Read the model definition and answer for the solid it produces. Units are mm, in the model's axes. Face numbers are marked on the shaded views. Give positions to 0.01 mm unless a question says otherwise; leave off trailing zeros. Order: outer loops, then holes, each group sorted by start corner. A loop starts at its lowest first (then second) coordinate and runs counter-clockwise, first axis right, second up.
```python
from build123d import *

# Parameters (mm, degrees)
F0_W     = 19.05
F0_H     = 152.4
F1_DEPTH = 6.35
F2_W     = 12.7
F2_H     = 152.4
F3_DEPTH = 5.08
F4_W     = 2.286
F4_H     = 3.81
F5_DEPTH = 152.4


with BuildPart() as f1:
    # F0 (on Top) → F1 (new body)
    with BuildSketch(Plane.XY):
        with Locations((-26.88839, 35.860999)):
            Rectangle(F0_W, F0_H)
    extrude(amount=F1_DEPTH)

    # F2 (on face) → F3 (cut)
    with BuildSketch(Plane.XY.offset(6.35)):
        with Locations((-26.903349, 35.860999)):
            Rectangle(F2_W, F2_H)
    extrude(amount=-F3_DEPTH, mode=Mode.SUBTRACT)

    # F4 (on face) → F5 (cut)
    with BuildSketch(Plane.XZ.offset(40.339001)):
        with Locations((-34.396349, 3.175)):
            Rectangle(F4_W, F4_H)
        with Locations((-19.410349, 3.175)):
            Rectangle(F4_W, F4_H)
    extrude(amount=-F5_DEPTH, mode=Mode.SUBTRACT)


solid = f1.part
```
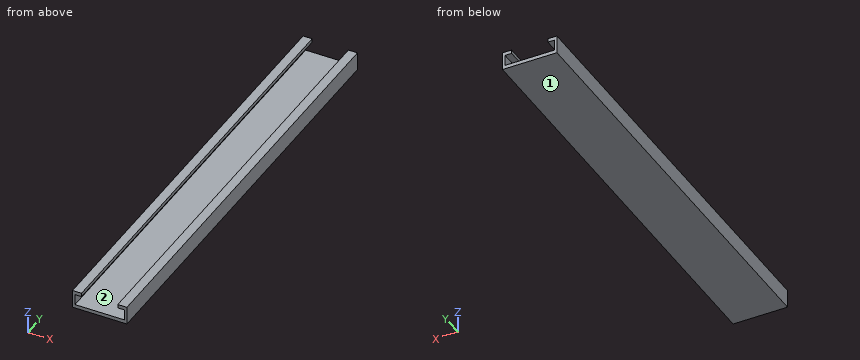
1) The part is cut by section C-C on x = -25.25. Determine the outline of the cut face in (y, z).
Final values:
outline: (-40.34, 0) - (112.06, 0) - (112.06, 1.27) - (-40.34, 1.27) - close
2) Consider L1, parallel to Z at x = -34.75, y = 49.5; L2, parallel to X at y = -12, z = 3.75; L3, parallel to Z at x = -26.25, y = 105. Determine where each line is inside the solid, lowest interval first.
Final values:
L1: z = 0 to 1.27, 5.08 to 6.35
L2: x = -36.41 to -35.54, -18.27 to -17.36
L3: z = 0 to 1.27
3) The part is cut by section B-B on y = 64. Determine the outline of the cut face in (x, z), and give its area (3 significant figures).
Final values:
outline: (-36.41, 0) - (-17.36, 0) - (-17.36, 6.35) - (-20.55, 6.35) - (-20.55, 5.08) - (-18.27, 5.08) - (-18.27, 1.27) - (-35.54, 1.27) - (-35.54, 5.08) - (-33.25, 5.08) - (-33.25, 6.35) - (-36.41, 6.35) - close
area: 39.0 mm2
4) For a pull along Z with two mould halves and no side action, classify the marked faces 1 and 2 as released by +Z, released by -Z, zero draft, split by the parting line, or undercut.
Final values:
face 1: released by -Z
face 2: undercut
5) Given pin 1 (2 mm diameter, centred on x = -34, z = 3, fed in from +Y), flat-ended and moving along its own axis, determine where the tip first touches the part or whether it passes through.
Final values:
pin 1: passes through
6) The part is cut by section A-A on z = 4. Determine the outline of the cut face in (x, y), and give its area (3 significant figures).
Final values:
outline: (-36.41, -40.34) - (-35.54, -40.34) - (-35.54, 112.06) - (-36.41, 112.06) - close; (-18.27, -40.34) - (-17.36, -40.34) - (-17.36, 112.06) - (-18.27, 112.06) - close
area: 271 mm2
